Work out the finished part from the listing and answer in its coordinate system (mm). Face numbers are marked on the shaded views. A direction names the side the tool comes from. Coordinates: 2 decimals unless noted, no trailing zeros. Order: outer loops, then holes, each group sorted by start corner. A loop starts at its lowest first (then second) coordinate and runs counter-clockwise, first axis right, second up. Notation, with made-up numbers: (48, 72.5) -> (61, 72.5) arc R29 ccw to (61, 108.5) -> close; hole circle Ø10 at (-40, 7). An arc over 180 degrees is marked (long way). Write item = value, one per line. Start each with the question number.
Q1. The part is cut by section A-A, the plane x = -40. Determine the outline of the cut face in (y, z).
Q2. The part is cut by section B-B, the plane y = 15. Determine the outline of the cut face in (x, z).
Q3. Which of the six approach directions +Z, -Z, +X, -X, +Y, -Y give full straight-line access (tool end or side, diameter ignored) to the marked faces 1 and 2?
Q4. The part is cut by section C-C, the plane z = 32. Determine the outline of the cut face in (x, y).
Q5. The part is cut by section D-D, the plane x = 0. Determine the outline of the cut face in (y, z).
Q6. For a pull along Y with two mould halves and no side action, classify the marked faces 3, 4 and 5 as +Y half, -Y half, draft (parallel to the pull), parting line (faces both ways), or undercut.
Q7. Straight lines are drawn through the part: L1, parallel to X at y = -0.95, z = 25; L2, parallel to Y at x = -22.75, z = 25; L3, parallel to Z at x = 22.75, y = 35. For each, find the intervals that lie inside material, in ascending order. Write a range as from..to.
Q8. Flat-ended cylindrical pins translate along their axes: pin 1 (5 mm diameter, centred on x = -15.5, z = 25, fed in from +Y); pin 2 (8 mm diameter, centred on y = 13.5, z = 23, fed in from -X); pin 3 (8 mm diameter, centred on x = -18, y = 27, fed in from -Z). Find the tip coordinate at first contact, or state that the pin passes through.
```python
from build123d import *

# Parameters (mm, degrees)
BOSS_EXTRUDE1_DEPTH = 50
CUT_EXTRUDE1_REACH  = 88.603
SKETCH2_R           = 3
SKETCH3_R           = 3
CUT_EXTRUDE2_DEPTH  = 70
FILLET2_RADIUS      = 25
FILLET2_LENGTH      = 1.5
FILLET3_RADIUS      = 25
FILLET3_LENGTH      = 1.5
SKETCH4_R           = 3
BOSS_EXTRUDE2_DEPTH = 5


with BuildPart() as part:
    # Sketch1 → Boss-Extrude1 (new body)
    with BuildSketch(Plane.XY):
        Polygon((50, -1.5), (-50, -1.5), (-50, 0), (-26.5, 0), (-26.5, 50), (-25, 50), (-25, 0), (25, 0), (25, 50), (26.5, 50), (26.5, 0), (50, 0), align=None)
    extrude(amount=BOSS_EXTRUDE1_DEPTH)

    # Sketch2 → Cut-Extrude1 (cut, up to next)
    with BuildSketch(Plane(origin=(0, 0, 0), x_dir=(1, 0, 0), z_dir=(0, 1, 0)), mode=Mode.PRIVATE) as cut_extrude1_sk1:
        with Locations(Location((-40, -25, 0), (0, 0, 270))):
            Circle(SKETCH2_R)
    cut_extrude1_tool1 = extrude(cut_extrude1_sk1.sketch, amount=-CUT_EXTRUDE1_REACH, mode=Mode.PRIVATE) & part.part
    # Sketch2 → Cut-Extrude1 (cut, up to next)
    with BuildSketch(Plane(origin=(0, 0, 0), x_dir=(1, 0, 0), z_dir=(0, 1, 0)), mode=Mode.PRIVATE) as cut_extrude1_sk2:
        with Locations(Location((40, -25, 0), (0, 0, 270))):
            Circle(SKETCH2_R)
    cut_extrude1_tool2 = extrude(cut_extrude1_sk2.sketch, amount=-CUT_EXTRUDE1_REACH, mode=Mode.PRIVATE) & part.part
    add(cut_extrude1_tool1.solids().sort_by_distance((-40, 0, 25))[0], mode=Mode.SUBTRACT)
    add(cut_extrude1_tool2.solids().sort_by_distance((40, 0, 25))[0], mode=Mode.SUBTRACT)

    # Sketch3 → Cut-Extrude2 (cut)
    with BuildSketch(Plane.ZY.offset(26.5)):
        with Locations(Location((25, 35, 0), (0, 0, 270))):
            Circle(SKETCH3_R)
    extrude(amount=-CUT_EXTRUDE2_DEPTH, mode=Mode.SUBTRACT)

    # Fillet2: full round fillet: the end face becomes a half cylinder, R = half its width
    fillet2_face = Plane((25.75, 50, 25), x_dir=(1, 0, 0), z_dir=(0, 1, 0))  # on the end face: x along it, z out of the body
    fillet2_slab = fillet2_face.offset(-FILLET2_RADIUS / 2) * Box(FILLET2_LENGTH, 2 * FILLET2_RADIUS, FILLET2_RADIUS, mode=Mode.PRIVATE)  # the body's end, R deep
    fillet2_round = Plane((25.75, 25, 25), x_dir=(0, 1, 0), z_dir=(1, 0, 0)) * Cylinder(FILLET2_RADIUS, FILLET2_LENGTH, mode=Mode.PRIVATE)  # its axis R under the face
    add(fillet2_slab - fillet2_round, mode=Mode.SUBTRACT)

    # Fillet3: full round fillet: the end face becomes a half cylinder, R = half its width
    fillet3_face = Plane((-25.75, 50, 25), x_dir=(-1, 0, 0), z_dir=(0, 1, 0))  # on the end face: x along it, z out of the body
    fillet3_slab = fillet3_face.offset(-FILLET3_RADIUS / 2) * Box(FILLET3_LENGTH, 2 * FILLET3_RADIUS, FILLET3_RADIUS, mode=Mode.PRIVATE)  # the body's end, R deep
    fillet3_round = Plane((-25.75, 25, 25), x_dir=(0, 1, 0), z_dir=(-1, 0, 0)) * Cylinder(FILLET3_RADIUS, FILLET3_LENGTH, mode=Mode.PRIVATE)  # its axis R under the face
    add(fillet3_slab - fillet3_round, mode=Mode.SUBTRACT)

    # Sketch4 → Boss-Extrude2 (add)
    with BuildSketch(Plane(origin=(-25, 0, 0), x_dir=(0, 0, -1), z_dir=(1, 0, 0))):
        Polygon((-30.196152423, 32), (-25, 29), (-19.803847577, 32), (-19.803847577, 38), (-25, 41), (-30.196152423, 38), align=None)
        with Locations(Location((-25, 35, 0), (0, 0, 270))):
            Circle(SKETCH4_R, mode=Mode.SUBTRACT)
    boss_extrude2 = extrude(amount=BOSS_EXTRUDE2_DEPTH)

    # Mirror1: Boss-Extrude2 across plane
    add(boss_extrude2.mirror(Plane(origin=(0, 0, 0), x_dir=(0, 0, 1), z_dir=(1, 0, 0))))


solid = part.part
```
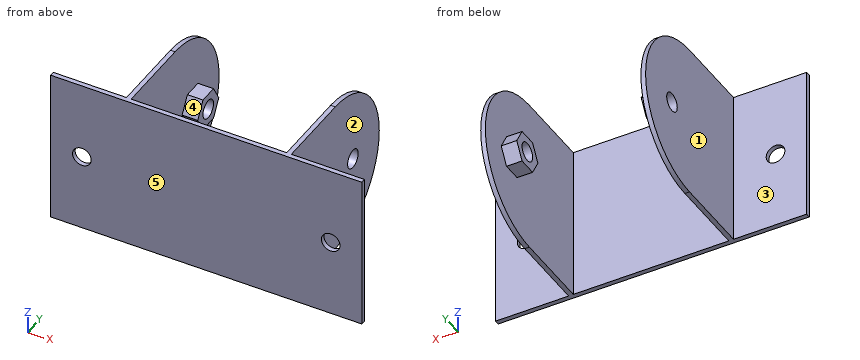
Model answer:
q1.outline = (-1.5, 0) -> (0, 0) -> (0, 22) -> (-1.5, 22) -> close; (-1.5, 28) -> (0, 28) -> (0, 50) -> (-1.5, 50) -> close
q2.outline = (-26.5, 0) -> (-25, 0) -> (-25, 50) -> (-26.5, 50) -> close; (25, 0) -> (26.5, 0) -> (26.5, 50) -> (25, 50) -> close
q3.face_1 = +Z, -Z, -X, +Y
q3.face_2 = +Z, -Z, +X, +Y
q4.outline = (-50, -1.5) -> (50, -1.5) -> (50, 0) -> (26.5, 0) -> (26.5, 49) -> (25, 49) -> (25, 0) -> (-25, 0) -> (-25, 49) -> (-26.5, 49) -> (-26.5, 0) -> (-50, 0) -> close
q5.outline = (-1.5, 0) -> (0, 0) -> (0, 50) -> (-1.5, 50) -> close
q6.face_3 = +Y half
q6.face_4 = undercut
q6.face_5 = -Y half
q7.L1 = -50..-43, -37..37, 43..50
q7.L2 = -1.5..0, 29..32, 38..41
q7.L3 = 19.8..22, 28..30.2
q8.pin_1 = 0
q8.pin_2 = -26.5
q8.pin_3 = 22.46
